```python
from build123d import *

# Parameters (mm, degrees)
SKETCH1_W           = 89.154
SKETCH1_H           = 35.56
BOSS_EXTRUDE1_DEPTH = 3.175
SKETCH2_W           = 3.2258
SKETCH2_H           = 6.35
CUT_EXTRUDE1_DEPTH  = 4.175
CUT_EXTRUDE2_DEPTH  = 4.175


with BuildPart() as part:
    # Sketch1 → Boss-Extrude1 (new body)
    with BuildSketch(Plane.XY):
        Rectangle(SKETCH1_W, SKETCH1_H)
    extrude(amount=BOSS_EXTRUDE1_DEPTH)

    # Sketch2 → Cut-Extrude1 (cut, through all)
    with BuildSketch(Plane.XY.offset(3.175)):
        with Locations((-36.6141, 9.525)):
            Rectangle(SKETCH2_W, SKETCH2_H)
        with Locations((-36.6141, -9.525)):
            Rectangle(SKETCH2_W, SKETCH2_H)
    cut_extrude1 = extrude(amount=-CUT_EXTRUDE1_DEPTH, mode=Mode.SUBTRACT)

    # Mirror1: Cut-Extrude1 across plane
    add(cut_extrude1.mirror(Plane(origin=(0, 0, 0), x_dir=(0, 0, 1), z_dir=(1, 0, 0))), mode=Mode.SUBTRACT)

    # Sketch3 → Cut-Extrude2 (cut, through all)
    with BuildSketch(Plane.XY.offset(3.175)):
        Polygon((-13.156260157, -11.43), (13.156260157, -11.43), (22.225, -17.78), (-22.225, -17.78), align=None)
    extrude(amount=-CUT_EXTRUDE2_DEPTH, mode=Mode.SUBTRACT)


solid = part.part
```
Source: CAD feature listing. Evaluate the final solid. Frame: model axes, mm. A direction names the side the tool comes from. Round coordinates to 2 decimals unless told otherwise and drop trailing zeros. Loops run counter-clockwise (first coordinate to the right, second up) from the corner with the lowest first, then second, coordinate; pieces in that order, holes last.
1. Section query D-D on x = 21. Output: boundary loops of the cut face in (y, z) (3 decimals), and give its area (3 significant figures).
2. Ray query, L1, parallel to X at y = -8.5, z = 0.3; L2, parallel to Y at x = -5.5, z = 0.45; L3, parallel to X at y = -11.5, z = 0.8. Return the intervals inside material, ascending.
3. Access query for faces 5 (the flat face through (37, 6.35, 2)), 6 (the flat face through (-1, 17.78, 2)), 7 (the flat face through (0, -11.43, 2)). Directions: +Z, -Z, +X, -X, +Y, -Y. A direction counts if a zero-diameter tool reaches every point of the face in a straight line with its end or side. Return the directions, or none.
4. Section query C-C on x = -4. Output: boundary loops of the cut face in (y, z) (3 decimals), and give its area (3 significant figures).
5. Contact query for a flat-ended pin moving along its axis: pin 1 (6 mm diameter, centred on x = -24.5, y = -12.5, fed in from -Z). Output: stop coordinate, or through.
6. Mould query, pull axis Y, two halves, no side actions, for faces 1 (the flat face through (-17.754, -14.649, 1.61)), 2 (the flat face through (-1, 0, 0)), 3 (the flat face through (-37, 12.7, 2)), 4 (the flat face through (-38.227, -10, 2)). Classes: released by +Y, released by -Y, zero draft, split by the parting line, or undercut.
7. Section query A-A on y = 9. Output: boundary loops of the cut face in (x, z) (3 decimals), and give its area (3 significant figures).
8. Section query B-B on z = 1.45. Output: boundary loops of the cut face in (x, y) (3 decimals), and give its area (3 significant figures).
Answers below:
1. outline: (-16.922, 0) - (17.78, 0) - (17.78, 3.175) - (-16.922, 3.175) - close
1. area: 110 mm2
2. L1: x = -44.58 to -38.23, -35 to 35, 38.23 to 44.58
2. L2: y = -11.43 to 17.78
2. L3: x = -44.58 to -38.23, -35 to -13.26, 13.26 to 35, 38.23 to 44.58
3. face 5: +Z, -Z
3. face 6: +Z, -Z, +X, -X, +Y
3. face 7: +Z, -Z, -Y
4. outline: (-11.43, 0) - (17.78, 0) - (17.78, 3.175) - (-11.43, 3.175) - close
4. area: 92.7 mm2
5. pin 1: stops at z = 0
6. face 1: released by -Y
6. face 2: zero draft
6. face 3: undercut
6. face 4: undercut
7. outline: (-44.577, 0) - (-38.227, 0) - (-38.227, 3.175) - (-44.577, 3.175) - close; (-35.001, 0) - (35.001, 0) - (35.001, 3.175) - (-35.001, 3.175) - close; (38.227, 0) - (44.577, 0) - (44.577, 3.175) - (38.227, 3.175) - close
7. area: 263 mm2
8. outline: (-44.577, -17.78) - (-22.225, -17.78) - (-13.156, -11.43) - (13.156, -11.43) - (22.225, -17.78) - (44.577, -17.78) - (44.577, 17.78) - (-44.577, 17.78) - close; hole (-38.227, -12.7) - (-35.001, -12.7) - (-35.001, -6.35) - (-38.227, -6.35) - close; hole (-38.227, 6.35) - (-35.001, 6.35) - (-35.001, 12.7) - (-38.227, 12.7) - close; hole (35.001, -12.7) - (38.227, -12.7) - (38.227, -6.35) - (35.001, -6.35) - close; hole (35.001, 6.35) - (38.227, 6.35) - (38.227, 12.7) - (35.001, 12.7) - close
8. area: 2,860 mm2
